Part model, mm, in its own coordinate system. Face numbers are marked on the shaded views. A direction names the side the tool comes from. Give positions to 0.01 mm unless a question says otherwise; leave off trailing zeros. Order: outer loops, then holes, each group sorted by start corner. A loop starts at its lowest first (then second) coordinate and runs counter-clockwise, first axis right, second up.
from build123d import *

# Parameters (mm, degrees)
BOSS_EXTRUDE1_DEPTH = 18.8


with BuildPart() as part:
    # Sketch1 → Boss-Extrude1 (new body)
    with BuildSketch(Plane.XY):
        with BuildLine():
            Line((41.5, -20), (34.641016151, -20))
            ThreePointArc((34.641016151, -20), (0, -40), (-34.641016151, -20))
            Line((-34.641016151, -20), (-41.5, -20))
            Line((-41.5, -20), (-41.5, 10))
            Line((-41.5, 10), (-53, 10))
            Line((-53, 10), (-53, -20))
            Line((-53, -20), (-55, -20))
            Line((-55, -20), (-55, -27.212333234))
            Line((-55, -27.212333234), (-41.5, -27.212333234))
            ThreePointArc((-41.5, -27.212333234), (0, -49.626213638), (41.5, -27.212333234))
            Line((41.5, -27.212333234), (55, -27.212333234))
            Line((55, -27.212333234), (55, -20))
            Line((55, -20), (53, -20))
            Line((53, -20), (53, 10))
            Line((53, 10), (41.5, 10))
            Line((41.5, 10), (41.5, -20))
        make_face()
    extrude(amount=-BOSS_EXTRUDE1_DEPTH)


solid = part.part
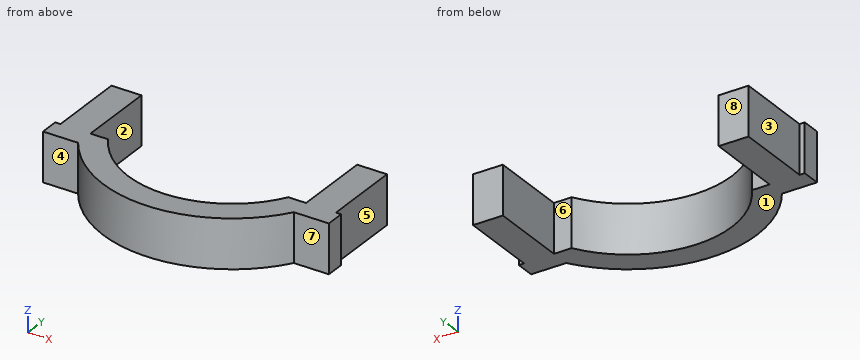
Item 1: Band-saw the part on B-B on z = -14. List the corners of the cut face in (x, y).
Item 2: Which spindle directions (+Z, -Z, +X, -X, +Y, -Y) get a long thin tool onto all of the face, cutting with end or side? Do the marked faces 4, 5, 6, 7 and 8. Say none if no direction does.
Item 3: Band-saw the part on C-C on y = -38. List the corners of the cut face in (x, z).
Item 4: Drill centre lines: probe 1 along X at (y, z) = (-9.5, -3.75); probe 2 along Y at (x, z) = (49.5, -9.5); probe 3 along X at (y, z) = (-35.5, -12.25). Where is each one in solid material? Low to high.
Item 5: Pull direction X, two halves, no side cores. Call the marked faces 1, 2 and 3: released by +X, released by -X, zero draft, split by the parting line, or undercut.
Item 6: Band-saw the part on A-A on y = -6. List the corners of the cut face in (x, z).
Item 7: Drop flat-ended pins along their axis: P1, Ø3.5, axis at x = -38.5, z = -13, coming from the +Y side; P2, Ø5, axis at x = -29.5, z = -11, coming from the +Y side; P3, Ø1.5, axis at x = 10.5, z = -5, coming from the -Y side; P4, Ø8, axis at y = -19.5, z = -2.5, coming from the +X side. Give the stop position or say it passes through.
Item 8: Band-saw the part on D-D on x = -31. List the corners of the cut face in (y, z), plus the area to 3 significant figures.
Working result:
1. outline: (-55, -27.21) - (-41.5, -27.21) arc R49.63 ccw to (41.5, -27.21) - (55, -27.21) - (55, -20) - (53, -20) - (53, 10) - (41.5, 10) - (41.5, -20) - (34.64, -20) arc R40 cw to (-34.64, -20) - (-41.5, -20) - (-41.5, 10) - (-53, 10) - (-53, -20) - (-55, -20) - close
2. face 4: +Z, -Z, -X, -Y
2. face 5: +Z, -Z, +X, +Y
2. face 6: +Z, -Z, +Y
2. face 7: +Z, -Z, +X, -Y
2. face 8: +Z, -Z, +X, -X, +Y
3. outline: (-31.92, -18.8) - (-12.49, -18.8) - (-12.49, 0) - (-31.92, 0) - close; (12.49, -18.8) - (31.92, -18.8) - (31.92, 0) - (12.49, 0) - close
4. probe 1: x = -53 to -41.5, 41.5 to 53
4. probe 2: y = -27.21 to 10
4. probe 3: x = -34.68 to -18.43, 18.43 to 34.68
5. face 1: zero draft
5. face 2: undercut
5. face 3: released by -X
6. outline: (-53, -18.8) - (-41.5, -18.8) - (-41.5, 0) - (-53, 0) - close; (41.5, -18.8) - (53, -18.8) - (53, 0) - (41.5, 0) - close
7. P1: stops at y = -20
7. P2: stops at y = -24
7. P3: stops at y = -48.66
7. P4: stops at x = 55
8. outline: (-38.75, -18.8) - (-25.28, -18.8) - (-25.28, 0) - (-38.75, 0) - close
8. area: 253 mm2
